```python
from build123d import *

# Parameters (mm, degrees)
F0_W     = 70.1
F0_H     = 142.3
F1_DEPTH = 8.1
F2_T     = -3
F3_R     = 2.99999


# Not quite as in the source:
# - a fillet or chamfer is up to 0.001 mm smaller than in the source, because OpenCascade refuses the exact size


with BuildPart() as f1:
    # F0 (on Top) → F1 (new body)
    with BuildSketch(Plane.XY):
        Rectangle(F0_W, F0_H)
    extrude(amount=F1_DEPTH)

    # F2
    f2_openings = [f1.faces().sort_by_distance(p)[0] for p in [
        (0, 0, 8.1),
    ]]
    offset(amount=F2_T, openings=f2_openings)

    # F3 (radius 3 in the source; OpenCascade refuses exactly that, so slightly less here)
    f3_edges = [f1.edges().sort_by_distance(p)[0] for p in [
        (-35.05, -71.15, 4.05),
        (35.05, -71.15, 4.05),
        (0, -71.15, 0),
        (0, -71.15, 8.1),
        (35.05, 71.15, 4.05),
        (35.05, 0, 0),
        (35.05, 0, 8.1),
        (-35.05, 71.15, 4.05),
        (0, 71.15, 0),
        (0, 71.15, 8.1),
        (-35.05, 0, 0),
        (-35.05, 0, 8.1),
    ]]
    fillet(f3_edges, radius=F3_R)


solid = f1.part
```
Verification items for the finished model (mm, model axes). A direction names the side the tool comes from. Round coordinates to 2 decimals unless told otherwise and drop trailing zeros. Order: outer loops, then holes, each group sorted by start corner. A loop starts at its lowest first (then second) coordinate and runs counter-clockwise, first axis right, second up. Notation, with made-up numbers: (54, 43) -> (62, 43) arc R20 ccw to (62, 51) -> close; hole circle Ø4 at (36, 8.5). An arc over 180 degrees is marked (long way). Put each result on its own line as item: value. Start each with the question number.
(1) Tool access check on faces 4 (the face through (0, -68.15, 6)), 5 (the face through (34.19, 0.95, 0.9)). Record the directions out of +Z, -Z, +X, -X, +Y, -Y that give a thin tool (end or side, any length) a straight path to the whole face; none if there is none.
(2) Section check C-C (z = 6.5). Enter the section's corners in (x, y).
(3) Draft check along X on faces 1 (the face through (0.45, -70.29, 7.2)), 2 (the face through (34.19, 70.25, 4.06)), 3 (the face through (0, 1, 3)). Enter one of: +X half, -X half, draft (parallel to the pull), parting line (faces both ways), or undercut.
(4) Material ranges on line 1 along Y through (x, z) = (32, 3.75); line 2 along X through (y, z) = (-36, 5.5); line 3 along Y through (x, z) = (-17, 5.5), recorded low to high.
(5) Depth check by flat-ended pin: pin 1 Ø4 at (x, z) = (-15.5, 6.5) entering from +Y; pin 2 Ø19 at (x, y) = (8.5, 27) entering from +Z; pin 3 Ø1.5 at (x, z) = (-15.5, 6) entering from -Y; pin 4 Ø1 at (y, z) = (-52, 1) entering from +X. Enter the tip coordinate at first touch or a pass-through.
Completed:
1. face 4: +Z
1. face 5: -Z, +X, +Y, -Y
2. outline: (-34.7, -68.15) arc R2.65 ccw to (-32.05, -70.8) -> (32.05, -70.8) arc R2.65 ccw to (34.7, -68.15) -> (34.7, 68.15) arc R2.65 ccw to (32.05, 70.8) -> (-32.05, 70.8) arc R2.65 ccw to (-34.7, 68.15) -> close; hole (-32.05, -68.15) -> (32.05, -68.15) -> (32.05, 68.15) -> (-32.05, 68.15) -> close
3. face 1: draft
3. face 2: +X half
3. face 3: undercut
4. line 1: y = -71.15 to -68.15, 68.15 to 71.15
4. line 2: x = -35.02 to -32.05, 32.05 to 35.02
4. line 3: y = -71.12 to -68.15, 68.15 to 71.12
5. pin 1: stops at y = 71.15
5. pin 2: stops at z = 3
5. pin 3: stops at y = -71.15
5. pin 4: stops at x = 34.65
